The figure shows three views and two pictorial views of one solid part (mm, origin at its lowest corner). Answer the questions. A direction names the side the tool comes from. Give positions to 0.01 mm unless a question says otherwise; leave off trailing zeros. Write each loop counter-clockwise with the first axis right and the second up, starting at its lowest first coordinate (ties: lowest second). Pieces come first, ordered by that corner, then holes. Notation, with made-up numbers: (30, -38) -> (66, -38) arc R18 cw to (66, -22) -> close; hole circle Ø2 at (70, -12.75). An arc over 180 degrees is marked (long way). Use a Markdown table: item, result.
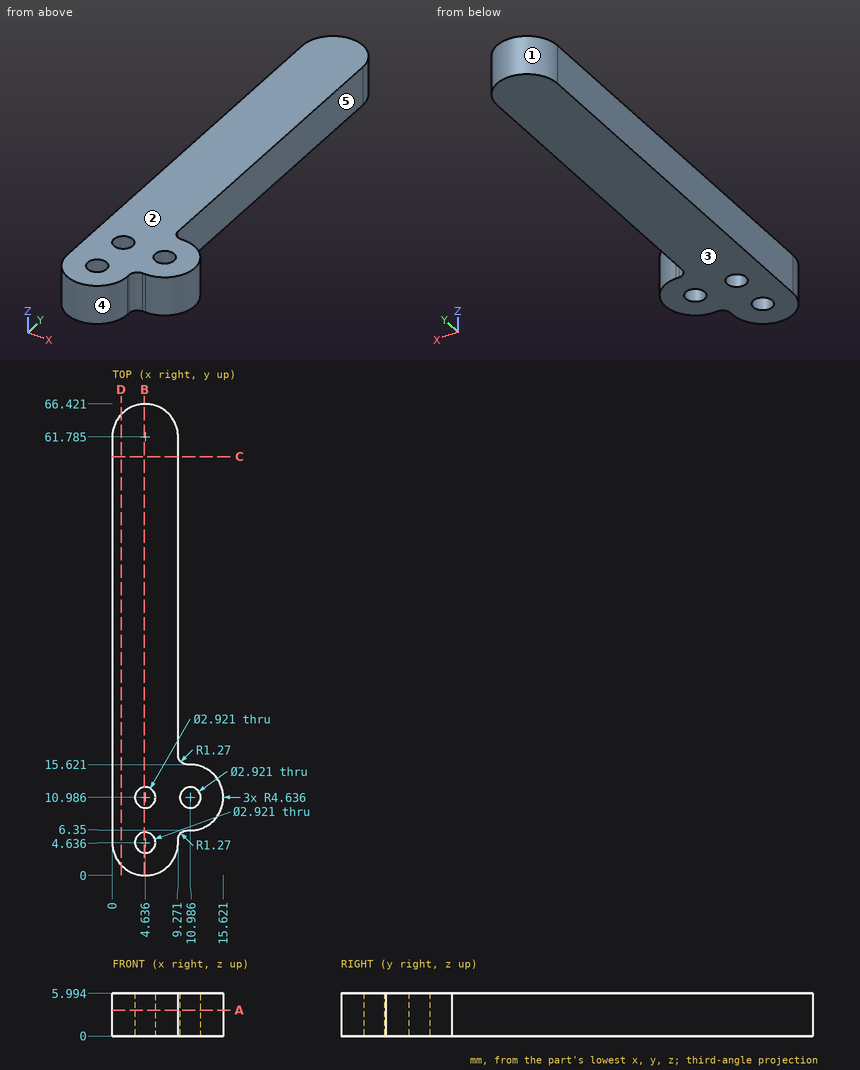
Item 1: For a pull along Z with two mould halves and no side action, classify the marked faces 1, 2 and 3 as +Z half, -Z half, draft (parallel to the pull), parting line (faces both ways), or undercut.
Return value:
| item | result |
|---|---|
| face 1 | draft |
| face 2 | +Z half |
| face 3 | -Z half |
Item 2: Straight lines are drawn through the part: line 1 along Y through (x, z) = (4.5, 5); line 2 along X through (y, z) = (18, 0.4); line 3 along Y through (x, z) = (11.5, 1.25). For each, find the intervals that lie inside material, in ascending order. Write a range as [from, to].
Return value:
| item | result |
|---|---|
| line 1 | [0, 3.18], [6.09, 9.53], [12.44, 66.42] |
| line 2 | [0, 9.27] |
| line 3 | [6.38, 9.62], [12.35, 15.59] |
Item 3: Each of these flat-tipped pins is pushed along its axis until it touches: P1, Ø1, axis at x = 8.5, y = 36, coming from the -Z side; P2, Ø0.5, axis at x = 11, z = 2.5, coming from the +Y side; P3, Ø0.5, axis at x = 10.5, z = 1.5, coming from the -Y side; P4, Ø1.5, axis at y = 23.5, z = 3.5, coming from the +X side. Where does it stop, or does it pass through?
Return value:
| item | result |
|---|---|
| P1 | z = 0 |
| P2 | y = 15.62 |
| P3 | y = 6.32 |
| P4 | x = 9.27 |
Item 4: A cutting plane is placed at C-C (y = 59). Give the vertices of the cut face in (x, z) (1 decimal).
Return value:
| item | result |
|---|---|
| outline | (0, 0) -> (9.3, 0) -> (9.3, 6) -> (0, 6) -> close |
Item 5: A tool of negligible diameter and unlimited length cuts with its end or side. For the marked faces 4 and 5, from which of +Z, -Z, +X, -X, +Y, -Y can it reach the whole face along a straight path? Write none if from no direction.
Return value:
| item | result |
|---|---|
| face 4 | +Z, -Z, -Y |
| face 5 | +Z, -Z, +X, +Y |
Item 6: A cutting plane is placed at B-B (x = 4.5). Give the vertices of the cut face in (y, z) (1 decimal), then the cut area to 3 significant figures.
Return value:
| item | result |
|---|---|
| outline | (0, 0) -> (3.2, 0) -> (3.2, 6) -> (0, 6) -> close; (6.1, 0) -> (9.5, 0) -> (9.5, 6) -> (6.1, 6) -> close; (12.4, 0) -> (66.4, 0) -> (66.4, 6) -> (12.4, 6) -> close |
| area | 363 mm^2 |
Item 7: A cutting plane is placed at D-D (x = 1.25). Give the vertices of the cut face in (y, z) (1 decimal).
Return value:
| item | result |
|---|---|
| outline | (1.5, 0) -> (65, 0) -> (65, 6) -> (1.5, 6) -> close |
Item 8: A cutting plane is placed at A-A (z = 3.65). Count the separate pieces of the cut face and the enclosed holes in it.
Return value:
| item | result |
|---|---|
| separate pieces | 1 |
| enclosed holes | 3 |
